from build123d import *

# Parameters (mm, degrees)
BOSS_EXTRUDE1_DEPTH  = 114.3
CUT_EXTRUDE1_START   = -1
SKETCH2_R            = 4
CUT_EXTRUDE1_DEPTH   = 7.35
M4_CLEARANCE_HOLE1_D = 4.5
FILLET1_R            = 4.7625


with BuildPart() as part:
    # Sketch1 → Boss-Extrude1 (new body)
    with BuildSketch(Plane(origin=(0, 0, 0), x_dir=(0, 0, -1), z_dir=(1, 0, 0))):
        with BuildLine():
            Line((0, 22.225), (-4, 22.225))
            Line((-4, 22.225), (-4, 15.839643355))
            ThreePointArc((-4, 15.839643355), (-2.015394761, 16.212109226), (0, 16.3369))
            Line((0, 16.3369), (0, 17.4625))
            Line((0, 17.4625), (0, 22.225))
        make_face()
        with BuildLine():
            ThreePointArc((0, 16.3369), (-2.015394761, 16.212109226), (-4, 15.839643355))
            ThreePointArc((-4, 15.839643355), (-16.3369, 0), (-4, -15.839643355))
            ThreePointArc((-4, -15.839643355), (-2.015394761, -16.212109226), (0, -16.3369))
            Line((0, -16.3369), (0, -12.5269))
            ThreePointArc((0, -12.5269), (-12.361865073, -2.026700652), (-4, 11.871108778))
            ThreePointArc((-4, 11.871108778), (-2.026700652, 12.361865073), (0, 12.5269))
            Line((0, 12.5269), (0, 16.3369))
        make_face()
        with BuildLine():
            ThreePointArc((0, -16.3369), (-2.015394761, -16.212109226), (-4, -15.839643355))
            Line((-4, -15.839643355), (-4, -22.225))
            Line((-4, -22.225), (0, -22.225))
            Line((0, -22.225), (0, -17.4625))
            Line((0, -17.4625), (0, -16.3369))
        make_face()
    extrude(amount=BOSS_EXTRUDE1_DEPTH)

    # Sketch2 → Cut-Extrude1 (cut)
    with BuildSketch(Plane.XY.offset(4).offset(CUT_EXTRUDE1_START)):
        with Locations((19.05, -17.37595)):
            Circle(SKETCH2_R)
        with Locations((57.15, -17.37595)):
            Circle(SKETCH2_R)
        with Locations((95.25, -17.37595)):
            Circle(SKETCH2_R)
    cut_extrude1 = extrude(amount=CUT_EXTRUDE1_DEPTH, mode=Mode.SUBTRACT)

    # M4 Clearance Hole1 (through all)
    with Locations(Plane.XY.offset(4)):
        with Locations((19.05, -17.37595), (57.15, -17.37595), (95.25, -17.37595)):
            m4_clearance_hole1 = Hole(M4_CLEARANCE_HOLE1_D / 2)

    # Mirror1: Cut-Extrude1, M4 Clearance Hole1 across plane
    add(cut_extrude1.mirror(Plane.ZX), mode=Mode.SUBTRACT)
    add(m4_clearance_hole1.mirror(Plane.ZX), mode=Mode.SUBTRACT)

    # Fillet1
    fillet1_edges = [part.edges().sort_by_distance(p)[0] for p in [
        (0, 22.225, 2),
        (0, -22.225, 2),
        (114.3, -22.225, 2),
        (114.3, 22.225, 2),
    ]]
    fillet(fillet1_edges, radius=FILLET1_R)


solid = part.part
The model under review builds one solid part; all positions refer to its coordinate system, in mm. A direction names the side the tool comes from. Round coordinates to 2 decimals unless told otherwise and drop trailing zeros. Order: outer loops, then holes, each group sorted by start corner. A loop starts at its lowest first (then second) coordinate and runs counter-clockwise, first axis right, second up. Notation, with made-up numbers: (7.5, 68) -> (35.5, 68) arc R19 ccw to (35.5, 93) -> close; hole circle Ø1 at (59.25, 23). An arc over 180 degrees is marked (long way). Write item = value, one per line. Start each with the question number.
Item 1: Consider section A-A on x = 19.05. Write out the cut boundary in (y, z) (3 decimals), plus the area to 3 significant figures.
Item 2: Consider section D-D on y = 6.5. Write out the cut boundary in (x, z), plus the area to 3 significant figures.
Item 3: For faces 4 (the face through (19.341, 13.387, 4.757)), 5 (the face through (56.35, 0.303, 16.334)), list the 3-axis set-ups (+Z, -Z, +X, -X, +Y, -Y) from which the entire face can be reached by the end or side of a thin tool; tool diameter is ignored.
Item 4: Consider section C-C on x = 76.5. Write out the cut boundary in (y, z) (3 decimals).
Item 5: For line 1 along Y through (x, z) = (57.15, 0.95) (3 decimals); line 2 along Y through (x, z) = (95.25, 1.4) (3 decimals); line 3 along Z through (x, y) = (45, -4), list the stretches that pass through material, from the lowest coordinate up.
Item 6: Consider section B-B on z = 5. Write out the cut boundary in (x, y).
Item 7: Clearance check with flat-ended pins moving along their axes: pin 1 Ø4 at (x, z) = (82, 6.5) entering from -Y; pin 2 Ø4 at (x, y) = (39, -2) entering from -Z; pin 3 Ø2.5 at (x, y) = (57, 19.5) entering from +Z. State where each tip first meets the part, or that it passes through.
Item 8: Mouldability with a two-part tool opening along X and no side actions: class faces 1 (the face through (57.441, -13.387, 4.757)), 2 (the face through (112.868, 20.867, 2.028)), 3 (the face through (56, -22.225, 2)) as released by +X, released by -X, zero draft, split by the parting line, or undercut.
Conclusion:
q1.outline = (-22.225, 0) -> (-19.626, 0) -> (-19.626, 3) -> (-21.376, 3) -> (-21.376, 4) -> (-22.225, 4) -> close; (-15.126, 0) -> (-12.527, 0) arc R12.527 cw to (12.527, 0) -> (15.126, 0) -> (15.126, 3) -> (13.376, 3) -> (13.376, 9.38) arc R16.337 ccw to (-13.376, 9.38) -> (-13.376, 3) -> (-15.126, 3) -> close; (19.626, 0) -> (22.225, 0) -> (22.225, 4) -> (21.376, 4) -> (21.376, 3) -> (19.626, 3) -> close
q1.area = 163 mm2
q2.outline = (0, 10.71) -> (114.3, 10.71) -> (114.3, 14.99) -> (0, 14.99) -> close
q2.area = 489 mm2
q3.face_4 = +Z
q3.face_5 = +Z, +X, -X
q4.outline = (-22.225, 0) -> (-12.527, 0) arc R12.527 cw to (12.527, 0) -> (22.225, 0) -> (22.225, 4) -> (15.84, 4) arc R16.337 ccw to (-15.84, 4) -> (-22.225, 4) -> close
q5.line_1 = -22.225 to -19.626, -15.126 to -12.491, 12.491 to 15.126, 19.626 to 22.225
q5.line_2 = -22.225 to -19.626, -15.126 to -12.448, 12.448 to 15.126, 19.626 to 22.225
q5.line_3 = 11.87 to 15.84
q6.outline = (0, -15.55) -> (15.49, -15.55) arc R4 cw to (22.61, -15.55) -> (53.59, -15.55) arc R4 cw to (60.71, -15.55) -> (91.69, -15.55) arc R4 cw to (98.81, -15.55) -> (114.3, -15.55) -> (114.3, -11.49) -> (0, -11.49) -> close; (0, 11.49) -> (114.3, 11.49) -> (114.3, 15.55) -> (98.81, 15.55) arc R4 cw to (91.69, 15.55) -> (60.71, 15.55) arc R4 cw to (53.59, 15.55) -> (22.61, 15.55) arc R4 cw to (15.49, 15.55) -> (0, 15.55) -> close
q7.pin_1 = -15.7
q7.pin_2 = 11.87
q7.pin_3 = 3
q8.face_1 = undercut
q8.face_2 = released by +X
q8.face_3 = zero draft
